Input: part model. Units: mm. Frame: model coordinates. Round coordinates to 2 decimals unless told otherwise and drop trailing zeros. Loops run counter-clockwise (first coordinate to the right, second up) from the corner with the lowest first, then second, coordinate; pieces in that order, holes last.
1) Section D-D, the plane y = 12. Return loops of the section in (x, z).
2) First-contact query: pin 1 (1 mm diameter, centred on x = -9.5, y = 17, fed in from +Z); pin 2 (2 mm diameter, centred on x = -5, y = 7.5, fed in from +Z); pin 3 (10 mm diameter, centred on y = 8.5, z = -7.5, fed in from +X). Flat tips, straight axial feed; report the tip coordinate or a pass-through.
3) Ray query, line 1 along Y through (x, z) = (-3.25, -0.25); line 2 along Y through (x, z) = (-0.25, 6.25); line 3 along X through (y, z) = (21, -10). Return the intervals inside material, ascending.
4) Section C-C, the plane x = -10.25. Return loops of the section in (y, z), and give its area (3 significant figures).
5) Section B-B, the plane y = 3. Return loops of the section in (x, z).
6) Section A-A, the plane z = 1.5. Return loops of the section in (x, y), and give its area (3 significant figures).
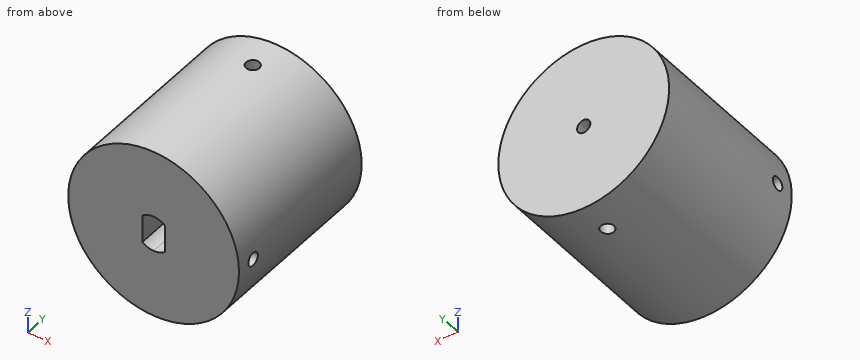
from build123d import *

# Parameters (mm, degrees)
SKETCH1_R               = 12.9
BOSS_EXTRUDE1_DEPTH     = 6
SKETCH2_R               = 12.9
BOSS_EXTRUDE2_DEPTH     = 20
SKETCH3_R               = 1
CUT_EXTRUDE2_DEPTH      = 5
SKETCH4_R               = 1
CUT_EXTRUDE3_DEPTH      = 18
CUT_EXTRUDE3_DEPTH_BACK = 19
CUT_EXTRUDE4_DEPTH      = 19
CUT_EXTRUDE4_DEPTH_BACK = 19
BOSS_EXTRUDE3_DEPTH     = 6
SKETCH7_R               = 1
CUT_EXTRUDE5_DEPTH      = 10


with BuildPart() as part:
    # Sketch1 → Boss-Extrude1 (new body)
    with BuildSketch(Plane(origin=(0, 0, 0), x_dir=(1, 0, 0), z_dir=(0, 1, 0))):
        with Locations((-0.136395343, 0.136395343)):
            Circle(SKETCH1_R)
        with BuildLine():
            Line((-2.036395343, -1.607164235), (-2.036395343, -2.054494887))
            ThreePointArc((-2.036395343, -2.054494887), (-1.150401835, -2.580549786), (-0.136395343, -2.763604657))
            ThreePointArc((-0.136395343, -2.763604657), (0.877611149, -2.580549786), (1.763604657, -2.054494887))
            Line((1.763604657, -2.054494887), (1.763604657, -1.607164235))
            Line((1.763604657, -1.607164235), (1.763604657, 1.87995492))
            Line((1.763604657, 1.87995492), (1.763604657, 2.327285573))
            ThreePointArc((1.763604657, 2.327285573), (0.877611149, 2.853340472), (-0.136395343, 3.036395343))
            ThreePointArc((-0.136395343, 3.036395343), (-1.150401835, 2.853340472), (-2.036395343, 2.327285573))
            Line((-2.036395343, 2.327285573), (-2.036395343, 1.87995492))
            Line((-2.036395343, 1.87995492), (-2.036395343, -1.607164235))
        make_face(mode=Mode.SUBTRACT)
    extrude(amount=BOSS_EXTRUDE1_DEPTH)

    # Sketch2 → Boss-Extrude2 (add)
    with BuildSketch(Plane(origin=(0, 6, 0), x_dir=(1, 0, 0), z_dir=(0, 1, 0))):
        with Locations((-0.136395343, 0.136395343)):
            Circle(SKETCH2_R)
    extrude(amount=BOSS_EXTRUDE2_DEPTH)

    # Sketch3 → Cut-Extrude2 (cut)
    with BuildSketch(Plane(origin=(0, 26, 0), x_dir=(1, 0, 0), z_dir=(0, 1, 0))):
        with Locations((-0.136395343, 0.136395343)):
            Circle(SKETCH3_R)
    extrude(amount=-CUT_EXTRUDE2_DEPTH, mode=Mode.SUBTRACT)

    # Sketch4 → Cut-Extrude3 (cut, two sides)
    with BuildSketch(Plane(origin=(0, 0, 0), x_dir=(0, 0, -1), z_dir=(1, 0, 0))) as cut_extrude3_sk:
        with Locations((0.136395343, 3)):
            Circle(SKETCH4_R)
    extrude(amount=CUT_EXTRUDE3_DEPTH, mode=Mode.SUBTRACT)
    extrude(cut_extrude3_sk.sketch, amount=-CUT_EXTRUDE3_DEPTH_BACK, mode=Mode.SUBTRACT)

    # Sketch5 → Cut-Extrude4 (cut, two sides)
    with BuildSketch(Plane.XY) as cut_extrude4_sk:
        with BuildLine():
            ThreePointArc((-1.136395343, 21), (-0.136395343, 20), (0.863604657, 21))
            Line((0.863604657, 21), (-1.136395343, 21))
        make_face()
        with BuildLine():
            Line((-1.136395343, 21), (0.863604657, 21))
            ThreePointArc((0.863604657, 21), (-0.136395343, 22), (-1.136395343, 21))
        make_face()
        with BuildLine():
            ThreePointArc((-1.136395343, 21), (-0.136395343, 20), (0.863604657, 21))
            Line((0.863604657, 21), (-1.136395343, 21))
        make_face()
        with BuildLine():
            Line((-1.136395343, 21), (0.863604657, 21))
            ThreePointArc((0.863604657, 21), (-0.136395343, 22), (-1.136395343, 21))
        make_face()
    extrude(amount=CUT_EXTRUDE4_DEPTH, mode=Mode.SUBTRACT)
    extrude(cut_extrude4_sk.sketch, amount=-CUT_EXTRUDE4_DEPTH_BACK, mode=Mode.SUBTRACT)

    # Sketch6 → Boss-Extrude3 (add)
    with BuildSketch(Plane.XZ):
        with BuildLine():
            ThreePointArc((-2.036395343, 2.054494887), (-0.136395343, 2.763604657), (1.763604657, 2.054494887))
            Line((1.763604657, 2.054494887), (1.763604657, -2.327285573))
            ThreePointArc((1.763604657, -2.327285573), (-0.136395343, -3.036395343), (-2.036395343, -2.327285573))
            Line((-2.036395343, -2.327285573), (-2.036395343, 2.054494887))
        make_face()
        with BuildLine():
            ThreePointArc((-0.136395343, 2.563604657), (-1.038180301, 2.408557287), (-1.836395343, 1.961222353))
            Line((-1.836395343, 1.961222353), (-1.836395343, 1.607164235))
            Line((-1.836395343, 1.607164235), (-1.836395343, -1.87995492))
            Line((-1.836395343, -1.87995492), (-1.836395343, -2.234013039))
            ThreePointArc((-1.836395343, -2.234013039), (-1.038180301, -2.681347973), (-0.136395343, -2.836395343))
            ThreePointArc((-0.136395343, -2.836395343), (0.765389615, -2.681347973), (1.563604657, -2.234013039))
            Line((1.563604657, -2.234013039), (1.563604657, -1.87995492))
            Line((1.563604657, -1.87995492), (1.563604657, 1.607164235))
            Line((1.563604657, 1.607164235), (1.563604657, 1.961222353))
            ThreePointArc((1.563604657, 1.961222353), (0.765389615, 2.408557287), (-0.136395343, 2.563604657))
        make_face(mode=Mode.SUBTRACT)
    extrude(amount=-BOSS_EXTRUDE3_DEPTH)

    # Sketch7 → Cut-Extrude5 (cut)
    with BuildSketch(Plane(origin=(0, 26, 0), x_dir=(1, 0, 0), z_dir=(0, 1, 0))):
        with Locations((-0.136395343, 0.136395343)):
            Circle(SKETCH7_R)
        with Locations((-0.136395343, 0.136395343)):
            Circle(SKETCH7_R)
    extrude(amount=-CUT_EXTRUDE5_DEPTH, mode=Mode.SUBTRACT)


solid = part.part
Final values:
1. outline: circle Ø25.8 at (-0.14, -0.14)
2. pin 1: stops at z = 9.24
2. pin 2: stops at z = 12.17
2. pin 3: stops at x = 12.55
3. line 1: y = 0 to 2.01, 3.99 to 26
3. line 2: y = 0 to 20.01, 21.99 to 26
3. line 3: x = -8.45 to -1.14, 0.86 to 8.18
4. outline: (0, -8.14) - (26, -8.14) - (26, 7.87) - (0, 7.87) - close; hole circle Ø2 at (3, -0.14)
4. area: 413 mm2
5. outline: (-13, -1.14) arc R12.9 ccw to (12.72, -1.14) - (1.76, -1.14) - (1.76, 0.86) - (12.72, 0.86) arc R12.9 ccw to (-13, 0.86) - (-2.04, 0.86) - (-2.04, -1.14) - close; hole (-1.84, -2.23) arc R2.7 ccw to (1.56, -2.23) - (1.56, 1.96) arc R2.7 ccw to (-1.84, 1.96) - close
6. outline: (-12.93, 0) - (-1.84, 0) - (-1.84, 6) - (1.56, 6) - (1.56, 0) - (12.66, 0) - (12.66, 26) - (-12.93, 26) - close; hole circle Ø2 at (-0.14, 21)
6. area: 642 mm2
